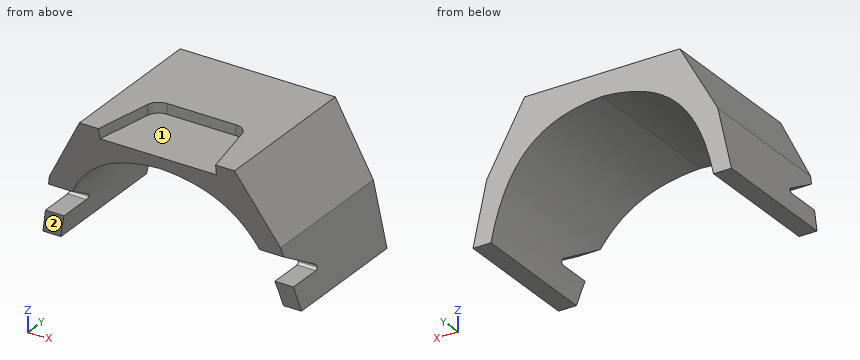
```python
from build123d import *

# Parameters (mm, degrees)
F1_DEPTH = 76.2
F3_DEPTH = 115.062
F5_DEPTH = 5.08
F7_DEPTH = 101.6
F9_DEPTH = 101.6


with BuildPart() as f1:
    # F0 (on Front) → F1 (new body)
    with BuildSketch(Plane.XZ):
        Polygon((38.1, 33.34175663), (0, 33.34175663), (-38.1, 33.34175663), (-56.7968450487, 0), (-63.5, -30.15824337), (0, -30.15824337), (63.5, -30.15824337), (56.7968450487, 0), align=None)
    extrude(amount=F1_DEPTH)

    # F2 (on face) → F3 (cut)
    with BuildSketch(Plane.XZ.offset(76.2)):
        with BuildLine():
            add(Edge.make_bspline(
                [(0, 22.3041530699), (29.2770247906, 20.8090394735), (46.7912144959, 7.9937791452), (54.6939596534, -30.15824337)],
                knots=[0, 0, 0, 0, 75.7874149366, 75.7874149366, 75.7874149366, 75.7874149366], degree=3))
            add(Edge.make_bspline(
                [(0, 22.3041530699), (-29.2770247906, 20.8090394735), (-46.7912144959, 7.9937791452), (-54.6939596534, -30.15824337)],
                knots=[0, 0, 0, 0, 75.7874149366, 75.7874149366, 75.7874149366, 75.7874149366], degree=3))
            Line((-54.6939596534, -30.15824337), (54.6939596534, -30.15824337))
        make_face()
    extrude(amount=-F3_DEPTH, mode=Mode.SUBTRACT)

    # F4 (on face) → F5 (cut)
    with BuildSketch(Plane.XY.offset(33.34175663)):
        with BuildLine():
            Line((-23.1831711448, -47.6289144868), (-28.7870969623, -76.2))
            Line((-28.7870969623, -76.2), (28.7870969623, -76.2))
            Line((28.7870969623, -76.2), (23.1831711448, -47.6289144868))
            ThreePointArc((23.1831711448, -47.6289144868), (20.9868440702, -43.9478771705), (16.9519010018, -42.5011143088))
            Line((16.9519010018, -42.5011143088), (0, -42.5011143088))
            Line((0, -42.5011143088), (-16.9519010018, -42.5011143088))
            ThreePointArc((-16.9519010018, -42.5011143088), (-20.9868440702, -43.9478771705), (-23.1831711448, -47.6289144868))
        make_face()
    extrude(amount=-F5_DEPTH, mode=Mode.SUBTRACT)

    # F6 (on Right) → F7 (cut, symmetric)
    with BuildSketch(Plane.YZ):
        with BuildLine():
            Line((-80.7253196836, 2.3729712702), (-78.2108455896, -18.6408273876))
            Line((-78.2108455896, -18.6408273876), (-49.9080079385, -18.6408273876))
            ThreePointArc((-49.9080079385, -18.6408273876), (-48.6147643972, -17.6525414948), (-49.2287055162, -16.1451383751))
            Line((-49.2287055162, -16.1451383751), (-80.7253196836, 2.3729712702))
        make_face()
    extrude(amount=F7_DEPTH, both=True, mode=Mode.SUBTRACT)

    # F8 (on Right) → F9 (cut, symmetric)
    with BuildSketch(Plane.YZ):
        Polygon((-85.8533158898, -35.2425277233), (-63.5725855827, -36.2190529704), (-76.2457847595, 33.6000360548), align=None)
    extrude(amount=F9_DEPTH, both=True, mode=Mode.SUBTRACT)


solid = f1.part
```
Model file for the job. Use its own axes, mm. Face numbers are marked on the shaded views. A direction names the side the tool comes from. Give positions to 0.01 mm unless a question says otherwise; leave off trailing zeros. One line per item, written item: value. Start each with the question number.
1. Probe L1, parallel to X at y = -39, z = -15; L2, parallel to X at y = -16, z = 12; L3, parallel to Z at x = -15, y = -71. List the from-to ranges inside material, lowest first. Write a range as from..to.
2. Which spindle directions (+Z, -Z, +X, -X, +Y, -Y) get a long thin tool onto all of the face, cutting with end or side? Do the marked faces 1 and 2. Say none if no direction does.
3. Pin check, flat tips, straight feed: pin 1 (8 mm diameter, centred on x = 49, y = -45.5, fed in from +Z); pin 2 (16.5 mm diameter, centred on x = -3.5, y = -67, fed in from +Z); pin 3 (2.5 mm diameter, centred on x = 55.5, y = -55, fed in from +Z); pin 4 (10 mm diameter, centred on x = -47, z = 23.5, fed in from +Y). Stop position of each tip, or through.
4. Slice it at A-A (y = -62). Give the number of separate pieces and of enclosed holes in the cut face, plus the area to 3 significant figures.
Solution:
1. L1: x = -60.13..-50.6, 50.6..60.13
1. L2: x = -50.07..-32.75, 32.75..50.07
1. L3: z = 20.24..28.26
2. face 1: +Z, -Y
2. face 2: -Z, +X, -X, -Y
3. pin 1: stops at z = 21.04
3. pin 2: stops at z = 28.26
3. pin 3: stops at z = 4.54
3. pin 4: stops at y = 0
4. separate pieces: 3
4. enclosed holes: 0
4. area: 1,920 mm^2
